Check sheet for the modelled part. Datum: model origin and axes. Units: mm. Face numbers are marked on the shaded views. A direction names the side the tool comes from. Coordinates: 2 decimals unless noted, no trailing zeros. Order: outer loops, then holes, each group sorted by start corner. A loop starts at its lowest first (then second) coordinate and runs counter-clockwise, first axis right, second up.
1. Draft check along X on the marked faces 1, 2 and 3. Enter one of: released by +X, released by -X, zero draft, split by the parting line, or undercut.
2. Thickness scan on line 1 (X direction, y = 0, z = 6.5); line 2 (Z direction, x = 15, y = -1); line 3 (Y direction, x = -10, z = 4.25). Record the ranges inside material, lowest first.
3. Set-up check for the marked faces 4 and 5: record each of +Z, -Z, +X, -X, +Y, -Y from which the full face is reachable in a straight line by a thin tool's end or side.
4. Cross-section at A-A (x = 46). Enter the section's corners in (y, z).
5. Cross-section at C-C (x = -58). Enter the section's corners in (y, z).
6. Cross-section at D-D (y = -15). Enter the section's corners in (x, z).
7. Gauge pin test, flat ends, axial feed: pin 1 Ø3 at (y, z) = (-9, 22) entering from -X; pin 2 Ø10 at (y, z) = (8, 18) entering from +X; pin 3 Ø10 at (x, z) = (-23.5, 6.5) entering from +Y. Record the tip position at first contact, or that the pin passes through.
```python
from build123d import *

# Parameters (mm, degrees)
F2_DEPTH = 12.7
F3_R     = 9.8806
F4_DEPTH = 12.7
F5_DEPTH = 12.7


# Not quite as in the source:
# - a variable given as a bare number and used for a length is read in inches; the dataset says mm whatever the document's units were


with BuildPart() as f2:
    # F1 (on Top) → F2 (new body)
    with BuildSketch(Plane.XY):
        with BuildLine():
            ThreePointArc((50.8, -16.9333333333), (65.8706666667, 0.9313333333), (48.006, 16.002))
            Line((48.006, 16.002), (-50.8, 16.002))
            ThreePointArc((-50.8, 16.002), (-67.2676666667, -0.4656666667), (-50.8, -16.9333333333))
            Line((-50.8, -16.9333333333), (50.8, -16.9333333333))
        make_face()
    extrude(amount=F2_DEPTH)

    # F3 (on face) → F4 (join)
    with BuildSketch(Plane.XY.offset(12.7)):
        with Locations((-50.8, -0.4656666667)):
            Circle(F3_R)
    extrude(amount=F4_DEPTH)

    # F3 (on face) → F5 (cut)
    with BuildSketch(Plane.XY.offset(12.7)):
        with Locations((49.403, -0.4656666667)):
            Circle(F3_R)
    extrude(amount=-F5_DEPTH, mode=Mode.SUBTRACT)


solid = f2.part
```
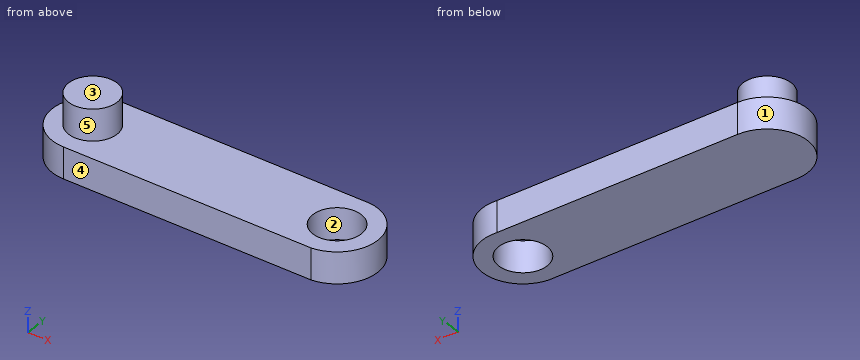
Data:
1. face 1: released by -X
1. face 2: undercut
1. face 3: zero draft
2. line 1: x = -67.26 to 39.53, 59.27 to 65.92
2. line 2: z = 0 to 12.7
2. line 3: y = -16.93 to 16
3. face 4: +Z, -Z, +X, -X, -Y
3. face 5: +Z
4. outline: (-16.93, 0) - (-9.74, 0) - (-9.74, 12.7) - (-16.93, 12.7) - close; (8.81, 0) - (16, 0) - (16, 12.7) - (8.81, 12.7) - close
5. outline: (-15.28, 0) - (14.34, 0) - (14.34, 12.7) - (6.3, 12.7) - (6.3, 25.4) - (-7.23, 25.4) - (-7.23, 12.7) - (-15.28, 12.7) - close
6. outline: (-58.54, 0) - (57.27, 0) - (57.27, 12.7) - (-58.54, 12.7) - close
7. pin 1: stops at x = -57.74
7. pin 2: stops at x = -41.55
7. pin 3: stops at y = 16
